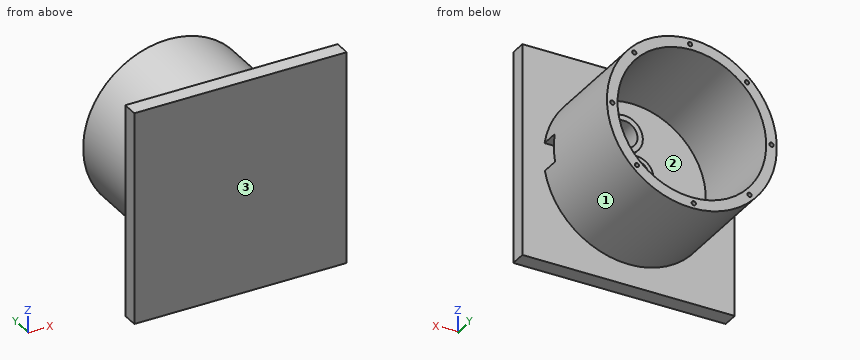
```python
from build123d import *

# Parameters (mm, degrees)
CROQUIS1_R              = 80
SALIENTE_EXTRUIR1_DEPTH = 5
CROQUIS2_R              = 80
CROQUIS2_R_2            = 70
SALIENTE_EXTRUIR2_DEPTH = 100
CROQUIS3_R              = 16.15
CROQUIS3_R_2            = 12.15
CROQUIS3_R_3            = 17.65
CROQUIS3_R_4            = 12.65
SALIENTE_EXTRUIR3_DEPTH = 8
SALIENTE_EXTRUIR4_DEPTH = 50
CROQUIS6_W              = 200
CROQUIS6_H              = 200
SALIENTE_EXTRUIR5_DEPTH = 15
CROQUIS8_W              = 26.192306131
CROQUIS8_H              = 16.90838964
CORTAR_EXTRUIR1_DEPTH   = 32
CROQUIS9_R              = 2
CORTAR_EXTRUIR2_DEPTH   = 10


with BuildPart() as part:
    # Croquis1 → Saliente-Extruir1 (new body)
    with BuildSketch(Plane(origin=(0, 0, 0), x_dir=(1, 0, 0), z_dir=(0, 1, 0))):
        with Locations(Location((0, 0, 0), (0, 0, 270))):
            Circle(CROQUIS1_R)
    extrude(amount=SALIENTE_EXTRUIR1_DEPTH)

    # Croquis2 → Saliente-Extruir2 (add)
    with BuildSketch(Plane(origin=(0, 5, 0), x_dir=(1, 0, 0), z_dir=(0, 1, 0))):
        with Locations(Location((0, 0, 0), (0, 0, 270))):
            Circle(CROQUIS2_R)
        with Locations(Location((0, 0, 0), (0, 0, 270))):
            Circle(CROQUIS2_R_2, mode=Mode.SUBTRACT)
    extrude(amount=SALIENTE_EXTRUIR2_DEPTH)

    # Croquis3 → Saliente-Extruir3 (add)
    # profile 1 of 2: a face of its own
    with BuildSketch(Plane(origin=(0, 5, 0), x_dir=(1, 0, 0), z_dir=(0, 1, 0))):
        with Locations(Location((0, 0, 0), (0, 0, 270))):
            Circle(CROQUIS3_R)
        with Locations(Location((0, 0, 0), (0, 0, 270))):
            Circle(CROQUIS3_R_2, mode=Mode.SUBTRACT)
    # profile 2 of 2: a face of its own
    with BuildSketch(Plane(origin=(0, 5, 0), x_dir=(1, 0, 0), z_dir=(0, 1, 0))):
        with Locations(Location((40, 0, 0), (0, 0, 270))):
            Circle(CROQUIS3_R_3)
        with Locations(Location((40, 0, 0), (0, 0, 270))):
            Circle(CROQUIS3_R_4, mode=Mode.SUBTRACT)
    extrude(amount=SALIENTE_EXTRUIR3_DEPTH)

    # Croquis5 → Saliente-Extruir4 (add)
    with BuildSketch(Plane(origin=(0, 13, 0), x_dir=(1, 0, 0), z_dir=(0, 1, 0))):
        with BuildLine():
            Line((50.235999238, 7.432820433), (56.008612695, 7.432820433))
            ThreePointArc((56.008612695, 7.432820433), (22.356299399, -0.471517861), (56.38275473, -6.567179567))
            Line((56.38275473, -6.567179567), (50.811783041, -6.567179567))
            ThreePointArc((50.811783041, -6.567179567), (27.360684958, -0.519822349), (50.235999238, 7.432820433))
        make_face()
    extrude(amount=SALIENTE_EXTRUIR4_DEPTH)

    # Croquis6 → Saliente-Extruir5 (add)
    with BuildSketch(Plane.XZ):
        Rectangle(CROQUIS6_W, CROQUIS6_H)
    extrude(amount=SALIENTE_EXTRUIR5_DEPTH)

    # Croquis8 → Cortar-Extruir1 (cut)
    with BuildSketch(Plane(origin=(100, 0, 0), x_dir=(0, 0, -1), z_dir=(1, 0, 0))):
        with Locations((0.906775278, 8.45419482)):
            Rectangle(CROQUIS8_W, CROQUIS8_H)
    extrude(amount=-CORTAR_EXTRUIR1_DEPTH, mode=Mode.SUBTRACT)

    # Croquis9 → Cortar-Extruir2 (cut)
    with BuildSketch(Plane(origin=(0, 105, 0), x_dir=(1, 0, 0), z_dir=(0, 1, 0))):
        with Locations(Location((-54.281139298, 51.78487788, 0), (0, 0, 270))):
            Circle(CROQUIS9_R)
        with Locations(Location((-1.765123376, 75, 0), (0, 0, 270))):
            Circle(CROQUIS9_R)
        with Locations(Location((-51.78487788, -54.281139298, 0), (0, 0, 270))):
            Circle(CROQUIS9_R)
        with Locations(Location((75, 1.765123376, 0), (0, 0, 270))):
            Circle(CROQUIS9_R)
        with Locations(Location((-75, -1.765123376, 0), (0, 0, 270))):
            Circle(CROQUIS9_R)
        with Locations(Location((1.765123376, -75, 0), (0, 0, 270))):
            Circle(CROQUIS9_R)
        with Locations(Location((54.281139298, -51.78487788, 0), (0, 0, 270))):
            Circle(CROQUIS9_R)
        with Locations(Location((51.78487788, 54.281139298, 0), (0, 0, 270))):
            Circle(CROQUIS9_R)
    extrude(amount=-CORTAR_EXTRUIR2_DEPTH, mode=Mode.SUBTRACT)


solid = part.part
```
Build history of the part. All positions in model axes, mm. Face numbers are marked on the shaded views. Coordinates: 2 decimals unless noted, no trailing zeros. Order: outer loops, then holes, each group sorted by start corner. A loop starts at its lowest first (then second) coordinate and runs counter-clockwise, first axis right, second up. Notation, with made-up numbers: M 5.5,73.5 L 63.5,73.5 A28 cw 63.5,110.5 Z; hole C 62.5,8.25 d10. An arc over 180 degrees is marked long. One line per question, with ' | ' between items. Start each with the question number.
1. Cut at C-C (y = 74). Write the cut outline in (x, z).
2. Cut at B-B (x = 40). Write the cut outline in (y, z), plus the area to 3 significant figures.
3. Mould opens along Z. For the marked faces 1, 2 and 3 say: +Z half, -Z half, draft (parallel to the pull), parting line (faces both ways), or undercut.
4. Flat gauge pins, fed straight in: P1, Ø6, axis at x = -17.5, z = 26, coming from the +Y side; P2, Ø10, axis at x = -40.5, y = 81.5, coming from the +Z side; P3, Ø1.5, axis at y = 15.5, z = 31, coming from the -X side. Where does each tip first touch, or does it go through?
5. Cut at A-A (y = 41). Write the cut outline in (x, z).
6. Wall check: line 1 along X through (y, z) = (39, 1); line 2 along Y through (x, z) = (-49.5, -84.5); line 3 along Y through (x, z) = (32, 6). Give the ranges that are in metal, low to high. Write a range as [from, to].
The answers:
1) outline: C 0,0 d160; hole C 0,0 d140
2) outline: M -15,-100 L 0,-100 L 0,-69.28 L 105,-69.28 L 105,-57.45 L 5,-57.45 L 5,-17.65 L 63,-17.65 L 63,-12.65 L 5,-12.65 L 5,12.65 L 63,12.65 L 63,17.65 L 5,17.65 L 5,57.45 L 105,57.45 L 105,69.28 L 0,69.28 L 0,100 L -15,100 Z | area: 6,640 mm2
3) face 1: parting line | face 2: undercut | face 3: draft
4) P1: stops at y = 5 | P2: stops at z = 71.69 | P3: stops at x = -74.06
5) outline: C 0,0 d160; M 50.24,-7.43 A12.65 cw long 50.81,6.57 L 56.38,6.57 A17.65 ccw long 56.01,-7.43 Z; hole C 0,0 d140
6) line 1: x = [-79.99, -69.99], [22.38, 27.39], [69.99, 79.99] | line 2: y = [-15, 0] | line 3: y = [-15, 5]
